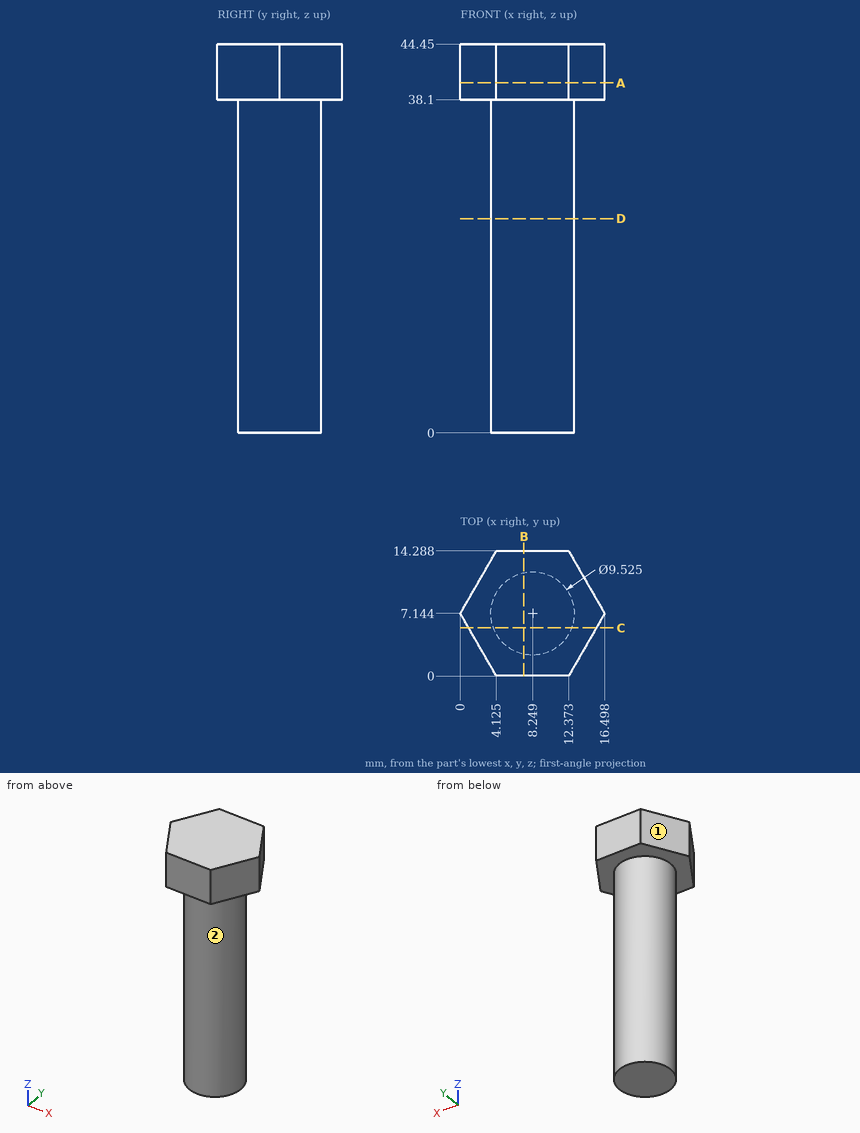
Drawing for the job (mm, zero at the part's lowest x, y, z). A direction names the side the tool comes from. Give positions to 0.01 mm unless a question says otherwise; leave off trailing zeros. Loops run counter-clockwise (first coordinate to the right, second up) from the corner with the lowest first, then second, coordinate; pieces in that order, holes last.
(1) Pin check, flat tips, straight feed: pin 1 (3 mm diameter, centred on y = 8.5, z = 30, fed in from +X); pin 2 (8 mm diameter, centred on x = 3.5, z = 20.5, fed in from -Y); pin 3 (5 mm diameter, centred on y = 4, z = 10, fed in from -X). Stop position of each tip, or through.
Return value:
pin 1: stops at x = 13.01
pin 2: stops at y = 2.44
pin 3: stops at x = 3.53
(2) Band-saw the part on B-B (x = 7.25). Write the cut outline in (y, z).
Return value:
outline: (0, 38.1) - (2.49, 38.1) - (2.49, 0) - (11.8, 0) - (11.8, 38.1) - (14.29, 38.1) - (14.29, 44.45) - (0, 44.45) - close
(3) Drill centre lines: line 1 along Y through (x, z) = (8.5, 32.5); line 2 along X through (y, z) = (7.25, 37.5); line 3 along Z through (x, y) = (1, 7.5). Where is each one in solid material? Low to high.
Return value:
line 1: y = 2.39 to 11.9
line 2: x = 3.49 to 13.01
line 3: z = 38.1 to 44.45
(4) Band-saw the part on D-D (z = 24.5). Write the cut outline in (x, y) (1 decimal).
Return value:
outline: circle Ø9.5 at (8.2, 7.1)
(5) Band-saw the part on A-A (z = 40). Write the cut outline in (x, y) (1 decimal).
Return value:
outline: (0, 7.1) - (4.1, 0) - (12.4, 0) - (16.5, 7.1) - (12.4, 14.3) - (4.1, 14.3) - close
(6) 3-axis set-ups, long thin cutter, end or side, ignore diameter. For the marked faces 1 and 2: which of +Z, -Z, +X, -X, +Y, -Y reach the whole face in a straight line?
Return value:
face 1: +Z, -Z, -X, +Y
face 2: -Z
(7) Band-saw the part on C-C (y = 5.5). Write the cut outline in (x, z), and give its area (3 significant figures).
Return value:
outline: (0.95, 38.1) - (3.78, 38.1) - (3.78, 0) - (12.72, 0) - (12.72, 38.1) - (15.55, 38.1) - (15.55, 44.45) - (0.95, 44.45) - close
area: 433 mm2
